The model under review builds one solid part; all positions refer to its coordinate system, in mm. A direction names the side the tool comes from. Round coordinates to 2 decimals unless told otherwise and drop trailing zeros. Order: outer loops, then holes, each group sorted by start corner. A loop starts at its lowest first (then second) coordinate and runs counter-clockwise, first axis right, second up.
```python
from build123d import *

# Parameters (mm, degrees)
BOSS_EXTRUDE1_DEPTH = 50.8
SKETCH3_R           = 2.4384
CUT_EXTRUDE1_DEPTH  = 103.556868279


with BuildPart() as part:
    # Sketch2 → Boss-Extrude1 (new body)
    with BuildSketch(Plane(origin=(0, 0, 0), x_dir=(1, 0, 0), z_dir=(0, 1, 0))):
        with BuildLine():
            Line((53.600169076, -6.35), (62.490169076, -6.35))
            Line((62.490169076, -6.35), (62.490169076, -9.525))
            Line((62.490169076, -9.525), (53.600169076, -9.525))
            Line((53.600169076, -9.525), (53.127911685, -9.525))
            ThreePointArc((53.127911685, -9.525), (-53.975, 0), (53.127911685, 9.525))
            Line((53.127911685, 9.525), (53.600169076, 9.525))
            Line((53.600169076, 9.525), (62.490169076, 9.525))
            Line((62.490169076, 9.525), (62.490169076, 6.35))
            Line((62.490169076, 6.35), (53.600169076, 6.35))
            Line((53.600169076, 6.35), (50.401562476, 6.35))
            ThreePointArc((50.401562476, 6.35), (-50.8, 0), (50.401562476, -6.35))
            Line((50.401562476, -6.35), (53.600169076, -6.35))
        make_face()
    extrude(amount=BOSS_EXTRUDE1_DEPTH)

    # Sketch3 → Cut-Extrude1 (cut, through all)
    with BuildSketch(Plane.XY.offset(9.525)):
        with Locations((58.292206061, 38.1)):
            Circle(SKETCH3_R)
        with Locations((58.292206061, 12.7)):
            Circle(SKETCH3_R)
    extrude(amount=-CUT_EXTRUDE1_DEPTH, mode=Mode.SUBTRACT)


solid = part.part
```
(1) Consider section B-B (y = 38.1). Write out the cut boundary in (x, z) (3 decimals), and give its area (3 significant figures).
Data:
outline: (50.402, -6.35) arc R50.8 cw (long way) to (50.402, 6.35) - (55.854, 6.35) - (55.854, 9.525) - (53.128, 9.525) arc R53.975 ccw (long way) to (53.128, -9.525) - (55.854, -9.525) - (55.854, -6.35) - close; (60.731, -9.525) - (62.49, -9.525) - (62.49, -6.35) - (60.731, -6.35) - close; (60.731, 6.35) - (62.49, 6.35) - (62.49, 9.525) - (60.731, 9.525) - close
area: 1,030 mm2
(2) Draft analysis for pull direction Y (two halves, no side actions). For faces 1 (the flat face through (17.5, 0, -48.2)), 2 (the cylindrical face through (59.42, 10.54, 7.96)), 3 (the flat face through (56, 25, 6.35)), state which applies: pulls with the +Y half, pulls with the -Y half, needs draft (parallel to the pull), parting line crosses it, or undercut.
Data:
face 1: pulls with the -Y half
face 2: undercut
face 3: needs draft
(3) To check wall thickness, follow probe 1 along Z at (x, y) = (56, 20) (3 decimals); probe 2 along Z at (x, y) = (45, 33); probe 3 along X at (y, z) = (34, 16.5). State the ranges of each line that lie inside material, in increasing order.
Data:
probe 1: z = -9.525 to -6.35, 6.35 to 9.525
probe 2: z = -29.8 to -23.57, 23.57 to 29.8
probe 3: x = -51.39 to -48.05, 48.05 to 51.39
(4) Consider section A-A (x = 0). Write out the cut boundary in (y, z) (3 decimals).
Data:
outline: (0, -53.975) - (50.8, -53.975) - (50.8, -50.8) - (0, -50.8) - close; (0, 50.8) - (50.8, 50.8) - (50.8, 53.975) - (0, 53.975) - close
(5) For faces 4 (the flat face through (58, 25, 9.525)), 5 (the flat face through (57, 25, -6.35)), 6 (the cylindrical face through (-53.93, 25.04, 2.24)), 7 (the cylindrical face through (57.975, 40.518, -7.915)), 8 (the flat face through (58, 25, -9.525)), list the 3-axis set-ups (+Z, -Z, +X, -X, +Y, -Y) from which the entire face can be reached by the end or side of a thin tool; tool diameter is ignored.
Data:
face 4: +Z, +X, +Y, -Y
face 5: +X, +Y, -Y
face 6: +Y, -Y
face 7: +Z, -Z
face 8: -Z, +X, +Y, -Y
(6) Consider section D-D (y = 20). Write out the cut boundary in (x, z) (3 decimals).
Data:
outline: (50.402, -6.35) arc R50.8 cw (long way) to (50.402, 6.35) - (62.49, 6.35) - (62.49, 9.525) - (53.128, 9.525) arc R53.975 ccw (long way) to (53.128, -9.525) - (62.49, -9.525) - (62.49, -6.35) - close
(7) Insertion check: pin 1 (4.5 mm diameter, centred on x = 60, y = 33, fed in from -Z) (3 decimals); pin 2 (2 mm diameter, centred on x = -21, y = 11.5, fed in from -Z); pin 3 (6 mm diameter, centred on y = 19, z = -7, fed in from -X). Each pin has a flat end and moves straight along its axis. Give the tip position at first contact, or say it passes through.
Data:
pin 1: stops at z = -9.525
pin 2: stops at z = -50.13
pin 3: stops at x = -53.83
(8) Consider section C-C (z = 46.5). Write out the cut boundary in (x, y).
Data:
outline: (-27.41, 0) - (-20.45, 0) - (-20.45, 50.8) - (-27.41, 50.8) - close; (20.45, 0) - (27.41, 0) - (27.41, 50.8) - (20.45, 50.8) - close
